from build123d import *

# Parameters (mm, degrees)
F0_R     = 4
F0_R_2   = 1.6
F1_DEPTH = 4


with BuildPart() as f1:
    # F0 (on Top) → F1 (new body)
    with BuildSketch(Plane.XY):
        with BuildLine():
            ThreePointArc((-44.464664, 71.088916), (-49.007351, 79.246936), (-51.001624, 88.369006))
            ThreePointArc((-51.001624, 88.369006), (-76.70394, 99.962521), (-72.157713, 72.135367))
            ThreePointArc((-72.157713, 72.135367), (-63.862626, 67.848082), (-57.158318, 61.348733))
            Line((-57.158318, 61.348733), (-28.612693, 24.147351))
            ThreePointArc((-28.612693, 24.147351), (-23.698236, 14.953048), (-22, 4.666985))
            Line((-22, 4.666985), (-22, -4.666985))
            ThreePointArc((-22, -4.666985), (-23.698236, -14.953048), (-28.612693, -24.147351))
            Line((-28.612693, -24.147351), (-57.158318, -61.348733))
            ThreePointArc((-57.158318, -61.348733), (-63.862626, -67.848082), (-72.157713, -72.135367))
            ThreePointArc((-72.157713, -72.135367), (-76.70394, -99.962521), (-51.001624, -88.369006))
            ThreePointArc((-51.001624, -88.369006), (-49.007351, -79.246936), (-44.464664, -71.088916))
            Line((-44.464664, -71.088916), (-25.387307, -46.22682))
            ThreePointArc((-25.387307, -46.22682), (0, -33.707185), (25.387307, -46.22682))
            Line((25.387307, -46.22682), (44.464664, -71.088916))
            ThreePointArc((44.464664, -71.088916), (49.007351, -79.246936), (51.001624, -88.369006))
            ThreePointArc((51.001624, -88.369006), (76.70394, -99.962521), (72.157713, -72.135367))
            ThreePointArc((72.157713, -72.135367), (63.862626, -67.848082), (57.158318, -61.348733))
            Line((57.158318, -61.348733), (28.612693, -24.147351))
            ThreePointArc((28.612693, -24.147351), (23.698236, -14.953048), (22, -4.666985))
            Line((22, -4.666985), (22, 4.666985))
            ThreePointArc((22, 4.666985), (23.698236, 14.953048), (28.612693, 24.147351))
            Line((28.612693, 24.147351), (57.158318, 61.348733))
            ThreePointArc((57.158318, 61.348733), (63.862626, 67.848082), (72.157713, 72.135367))
            ThreePointArc((72.157713, 72.135367), (76.70394, 99.962521), (51.001624, 88.369006))
            ThreePointArc((51.001624, 88.369006), (49.007351, 79.246936), (44.464664, 71.088916))
            Line((44.464664, 71.088916), (23.817164, 44.18057))
            ThreePointArc((23.817164, 44.18057), (20.72098, 42.300752), (17.167911, 43.004867))
            ThreePointArc((17.167911, 43.004867), (0, 48), (-17.167911, 43.004867))
            ThreePointArc((-17.167911, 43.004867), (-20.72098, 42.300752), (-23.817164, 44.18057))
            Line((-23.817164, 44.18057), (-44.464664, 71.088916))
        make_face()
        with BuildLine():
            ThreePointArc((-67.701649, -93.922101), (-66.324179, -92.126947), (-64.529025, -93.504417))
            Line((-64.529025, -93.504417), (-64.111341, -96.677041))
            ThreePointArc((-64.111341, -96.677041), (-65.488811, -98.472194), (-67.283965, -97.094724))
            Line((-67.283965, -97.094724), (-67.701649, -93.922101))
        make_face(mode=Mode.SUBTRACT)
        with BuildLine():
            Line((-73.199307, -89.703599), (-76.37193, -90.121283))
            ThreePointArc((-76.37193, -90.121283), (-78.167084, -88.743813), (-76.789614, -86.94866))
            Line((-76.789614, -86.94866), (-73.616991, -86.530976))
            ThreePointArc((-73.616991, -86.530976), (-71.821837, -87.908446), (-73.199307, -89.703599))
        make_face(mode=Mode.SUBTRACT)
        with Locations((-66.963757, -87.268867)):
            Circle(F0_R, mode=Mode.SUBTRACT)
        with BuildLine():
            Line((-66.643549, -77.44301), (-66.225866, -80.615634))
            ThreePointArc((-66.225866, -80.615634), (-67.603336, -82.410788), (-69.398489, -81.033318))
            Line((-69.398489, -81.033318), (-69.816173, -77.860694))
            ThreePointArc((-69.816173, -77.860694), (-68.438703, -76.06554), (-66.643549, -77.44301))
        make_face(mode=Mode.SUBTRACT)
        with BuildLine():
            ThreePointArc((-60.310524, -88.006759), (-62.105677, -86.629289), (-60.728207, -84.834135))
            Line((-60.728207, -84.834135), (-57.555584, -84.416452))
            ThreePointArc((-57.555584, -84.416452), (-55.76043, -85.793921), (-57.1379, -87.589075))
            Line((-57.1379, -87.589075), (-60.310524, -88.006759))
        make_face(mode=Mode.SUBTRACT)
        with Locations((-18, -28)):
            Circle(F0_R_2, mode=Mode.SUBTRACT)
        with Locations((-15.25, -15.25)):
            Circle(F0_R_2, mode=Mode.SUBTRACT)
        with BuildLine():
            ThreePointArc((60.728207, -84.834135), (62.105677, -86.629289), (60.310524, -88.006759))
            Line((60.310524, -88.006759), (57.1379, -87.589075))
            ThreePointArc((57.1379, -87.589075), (55.76043, -85.793921), (57.555584, -84.416452))
            Line((57.555584, -84.416452), (60.728207, -84.834135))
        make_face(mode=Mode.SUBTRACT)
        with BuildLine():
            ThreePointArc((64.529025, -93.504417), (66.324179, -92.126947), (67.701649, -93.922101))
            Line((67.701649, -93.922101), (67.283965, -97.094724))
            ThreePointArc((67.283965, -97.094724), (65.488811, -98.472194), (64.111341, -96.677041))
            Line((64.111341, -96.677041), (64.529025, -93.504417))
        make_face(mode=Mode.SUBTRACT)
        with Locations((66.963757, -87.268867)):
            Circle(F0_R, mode=Mode.SUBTRACT)
        with BuildLine():
            Line((69.816173, -77.860694), (69.398489, -81.033318))
            ThreePointArc((69.398489, -81.033318), (67.603336, -82.410788), (66.225866, -80.615634))
            Line((66.225866, -80.615634), (66.643549, -77.44301))
            ThreePointArc((66.643549, -77.44301), (68.438703, -76.06554), (69.816173, -77.860694))
        make_face(mode=Mode.SUBTRACT)
        with BuildLine():
            Line((76.37193, -90.121283), (73.199307, -89.703599))
            ThreePointArc((73.199307, -89.703599), (71.821837, -87.908446), (73.616991, -86.530976))
            Line((73.616991, -86.530976), (76.789614, -86.94866))
            ThreePointArc((76.789614, -86.94866), (78.167084, -88.743813), (76.37193, -90.121283))
        make_face(mode=Mode.SUBTRACT)
        with Locations((18, -28)):
            Circle(F0_R_2, mode=Mode.SUBTRACT)
        with Locations((15.25, -15.25)):
            Circle(F0_R_2, mode=Mode.SUBTRACT)
        with BuildLine():
            Line((-18.5, -10.5), (-18.5, 10.5))
            ThreePointArc((-18.5, 10.5), (-17.25, 11.75), (-16, 10.5))
            Line((-16, 10.5), (-16, -10.5))
            ThreePointArc((-16, -10.5), (-17.25, -11.75), (-18.5, -10.5))
        make_face(mode=Mode.SUBTRACT)
        with Locations((-15.25, 15.25)):
            Circle(F0_R_2, mode=Mode.SUBTRACT)
        with Locations((-18, 37)):
            Circle(F0_R_2, mode=Mode.SUBTRACT)
        with BuildLine():
            Line((-76.37193, 90.121283), (-73.199307, 89.703599))
            ThreePointArc((-73.199307, 89.703599), (-71.821837, 87.908446), (-73.616991, 86.530976))
            Line((-73.616991, 86.530976), (-76.789614, 86.94866))
            ThreePointArc((-76.789614, 86.94866), (-78.167084, 88.743813), (-76.37193, 90.121283))
        make_face(mode=Mode.SUBTRACT)
        with BuildLine():
            Line((-69.816173, 77.860694), (-69.398489, 81.033318))
            ThreePointArc((-69.398489, 81.033318), (-67.603336, 82.410788), (-66.225866, 80.615634))
            Line((-66.225866, 80.615634), (-66.643549, 77.44301))
            ThreePointArc((-66.643549, 77.44301), (-68.438703, 76.06554), (-69.816173, 77.860694))
        make_face(mode=Mode.SUBTRACT)
        with Locations((-66.963757, 87.268867)):
            Circle(F0_R, mode=Mode.SUBTRACT)
        with BuildLine():
            Line((-64.111341, 96.677041), (-64.529025, 93.504417))
            ThreePointArc((-64.529025, 93.504417), (-66.324179, 92.126947), (-67.701649, 93.922101))
            Line((-67.701649, 93.922101), (-67.283965, 97.094724))
            ThreePointArc((-67.283965, 97.094724), (-65.488811, 98.472194), (-64.111341, 96.677041))
        make_face(mode=Mode.SUBTRACT)
        with BuildLine():
            ThreePointArc((-60.728207, 84.834135), (-62.105677, 86.629289), (-60.310524, 88.006759))
            Line((-60.310524, 88.006759), (-57.1379, 87.589075))
            ThreePointArc((-57.1379, 87.589075), (-55.76043, 85.793921), (-57.555584, 84.416452))
            Line((-57.555584, 84.416452), (-60.728207, 84.834135))
        make_face(mode=Mode.SUBTRACT)
        with BuildLine():
            ThreePointArc((16, 10.5), (17.25, 11.75), (18.5, 10.5))
            Line((18.5, 10.5), (18.5, -10.5))
            ThreePointArc((18.5, -10.5), (17.25, -11.75), (16, -10.5))
            Line((16, -10.5), (16, 10.5))
        make_face(mode=Mode.SUBTRACT)
        with Locations((15.25, 15.25)):
            Circle(F0_R_2, mode=Mode.SUBTRACT)
        with Locations((18, 37)):
            Circle(F0_R_2, mode=Mode.SUBTRACT)
        with BuildLine():
            Line((57.1379, 87.589075), (60.310524, 88.006759))
            ThreePointArc((60.310524, 88.006759), (62.105677, 86.629289), (60.728207, 84.834135))
            Line((60.728207, 84.834135), (57.555584, 84.416452))
            ThreePointArc((57.555584, 84.416452), (55.76043, 85.793921), (57.1379, 87.589075))
        make_face(mode=Mode.SUBTRACT)
        with BuildLine():
            Line((66.643549, 77.44301), (66.225866, 80.615634))
            ThreePointArc((66.225866, 80.615634), (67.603336, 82.410788), (69.398489, 81.033318))
            Line((69.398489, 81.033318), (69.816173, 77.860694))
            ThreePointArc((69.816173, 77.860694), (68.438703, 76.06554), (66.643549, 77.44301))
        make_face(mode=Mode.SUBTRACT)
        with Locations((66.963757, 87.268867)):
            Circle(F0_R, mode=Mode.SUBTRACT)
        with BuildLine():
            Line((76.789614, 86.94866), (73.616991, 86.530976))
            ThreePointArc((73.616991, 86.530976), (71.821837, 87.908446), (73.199307, 89.703599))
            Line((73.199307, 89.703599), (76.37193, 90.121283))
            ThreePointArc((76.37193, 90.121283), (78.167084, 88.743813), (76.789614, 86.94866))
        make_face(mode=Mode.SUBTRACT)
        with BuildLine():
            Line((64.529025, 93.504417), (64.111341, 96.677041))
            ThreePointArc((64.111341, 96.677041), (65.488811, 98.472194), (67.283965, 97.094724))
            Line((67.283965, 97.094724), (67.701649, 93.922101))
            ThreePointArc((67.701649, 93.922101), (66.324179, 92.126947), (64.529025, 93.504417))
        make_face(mode=Mode.SUBTRACT)
    extrude(amount=F1_DEPTH)


solid = f1.part
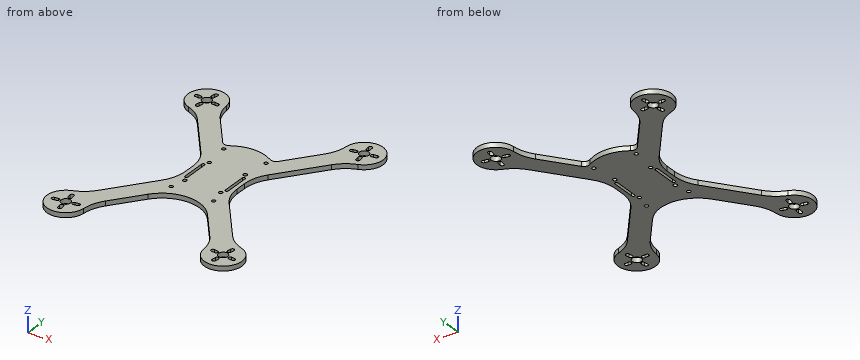
Read the model definition and answer for the solid it produces. Units are mm, in the model's axes. Coordinates: 2 decimals unless noted, no trailing zeros. Order: outer loops, then holes, each group sorted by start corner. A loop starts at its lowest first (then second) coordinate and runs counter-clockwise, first axis right, second up. Notation, with made-up numbers: (77.5, 6.25) -> (135.5, 6.25) arc R24 cw to (135.5, 22.25) -> close; hole circle Ø8 at (-6, 59.5). An arc over 180 degrees is marked (long way). Answer as a JSON object with one key per item and string values.
1) A cutting plane is placed at C-C, the plane y = 33. Determine the outline of the cut face in (x, z).
Model answer:
{"outline": "(-35.41, 0) -> (35.41, 0) -> (35.41, 4) -> (-35.41, 4) -> close"}
2) Each of these flat-tipped pins is pushed along its axis until it touches: pin 1 (2 mm diameter, centred on y = 54.5, z = 2.5, fed in from +X); pin 2 (1.2 mm diameter, centred on y = 3, z = 2.5, fed in from +X); pin 3 (2 mm diameter, centred on x = 41, z = 3.5, fed in from -Y); pin 4 (1.9 mm diameter, centred on x = 15.25, y = -15.25, fed in from +Z). Where does it stop, or does it pass through?
Model answer:
{"pin 1": "stops at x = 52.67", "pin 2": "stops at x = 22", "pin 3": "stops at y = -67.88", "pin 4": "passes through"}
3) A cutting plane is placed at A-A, the plane x = -47. Determine the outline of the cut face in (y, z), plus the area to 3 significant figures.
Model answer:
{"outline": "(-74.94, 0) -> (-48.11, 0) -> (-48.11, 4) -> (-74.94, 4) -> close; (48.11, 0) -> (74.94, 0) -> (74.94, 4) -> (48.11, 4) -> close", "area": "215 mm²"}
4) A cutting plane is placed at D-D, the plane x = -11. Determine the outline of the cut face in (y, z).
Model answer:
{"outline": "(-35.66, 0) -> (46.05, 0) -> (46.05, 4) -> (-35.66, 4) -> close"}
5) Consider line 1 along X through (y, z) = (6.5, 0.25); line 2 along Y through (x, z) = (-74.5, 3.4); line 3 along Y through (x, z) = (14.5, 3.15). Determine where each line is inside the solid, lowest interval first. Write a range as from..to.
Model answer:
{"line 1": "x = -22.05..-18.5, -16..16, 18.5..22.05", "line 2": "y = -101.38..-89.87, -86.65..-73.15, 73.15..86.65, 89.87..101.38", "line 3": "y = -37.18..-16.66, -13.84..13.84, 16.66..44.53"}
6) A cutting plane is placed at B-B, the plane z = 3.1. State how many separate pieces and enclosed holes the cut face has, plus the area to 3 significant figures.
Model answer:
{"separate pieces": "1", "enclosed holes": "30", "area": "10,100 mm²"}
